Can you work these out from the model? Positions are in its coordinate system, mm. Coordinates: 2 decimals unless noted, no trailing zeros. Order: outer loops, then holes, each group sorted by start corner. A loop starts at its lowest first (then second) coordinate and runs counter-clockwise, first axis right, second up. Notation, with made-up numbers: (13.25, 82) - (70.25, 82) arc R36 cw to (70.25, 118) - close; hole circle Ø7 at (-7, 50). An arc over 180 degrees is marked (long way). Return JSON: item names as keys, results as strings. Group by question number.
1) If I drill on line 1 along Y through (x, z) = (0, -1.15); line 2 along X through (y, z) = (6.5, -1.25); line 3 along Y through (x, z) = (-3.5, -2.6), over which ranges is the centre line in solid material (lowest first)?
2) Imagine slicing it at A-A (y = -20). Write out the boundary of the cut face in (x, z), and give its area (3 significant figures).
3) Imagine slicing it at D-D (y = -10). Write out the boundary of the cut face in (x, z).
4) Imagine slicing it at B-B (z = -0.75). Give the number of separate pieces and of enclosed holes in the cut face, and give its area (3 significant figures).
5) For pin 1 Ø9 at (x, y) = (0, -20) entering from -Z, with a flat end and sliding along its axis, tell me the tip position at first contact or that it passes through.
6) Imagine slicing it at C-C (x = 13). Write out the boundary of the cut face in (y, z), and give its area (3 significant figures).
```python
from build123d import *

# Parameters (mm, degrees)
SM_BASE_FLANGE_1_DEPTH = 3
CUT_EXTRUDE_1_REACH    = 41.166
SKETCH_6_R             = 2.5
CUT_EXTRUDE_2_REACH    = 41.166
SKETCH_7_R             = 5


# Sheet-metal steps are written as plain solids
with BuildPart() as part:
    # Sketch 1 → 基体-法兰1 (new body)
    with BuildSketch(Plane.XY):
        Polygon((20, -30), (14.284239003, -30), (-14.284239003, -30), (-20, -30), (-25, -25), (-25, 21.339745962), (-20, 30), (20, 30), (25, 21.339745962), (25, -25), align=None)
    extrude(amount=-SM_BASE_FLANGE_1_DEPTH)

    # 草图6 → 切除-拉伸1 (cut, up to next)
    with BuildSketch(Plane.XY, mode=Mode.PRIVATE) as cut_extrude_1_sk1:
        with Locations((0, 24)):
            Circle(SKETCH_6_R)
    cut_extrude_1_tool1 = extrude(cut_extrude_1_sk1.sketch, amount=-CUT_EXTRUDE_1_REACH, mode=Mode.PRIVATE) & part.part
    # 草图6 → 切除-拉伸1 (cut, up to next)
    with BuildSketch(Plane.XY, mode=Mode.PRIVATE) as cut_extrude_1_sk2:
        with Locations((-17.8, -10)):
            Circle(SKETCH_6_R)
    cut_extrude_1_tool2 = extrude(cut_extrude_1_sk2.sketch, amount=-CUT_EXTRUDE_1_REACH, mode=Mode.PRIVATE) & part.part
    # 草图6 → 切除-拉伸1 (cut, up to next)
    with BuildSketch(Plane.XY, mode=Mode.PRIVATE) as cut_extrude_1_sk3:
        with Locations((17.8, -10)):
            Circle(SKETCH_6_R)
    cut_extrude_1_tool3 = extrude(cut_extrude_1_sk3.sketch, amount=-CUT_EXTRUDE_1_REACH, mode=Mode.PRIVATE) & part.part
    # 草图6 → 切除-拉伸1 (cut, up to next)
    with BuildSketch(Plane.XY, mode=Mode.PRIVATE) as cut_extrude_1_sk4:
        with Locations((-12.5, 20)):
            Circle(SKETCH_6_R)
    cut_extrude_1_tool4 = extrude(cut_extrude_1_sk4.sketch, amount=-CUT_EXTRUDE_1_REACH, mode=Mode.PRIVATE) & part.part
    # 草图6 → 切除-拉伸1 (cut, up to next)
    with BuildSketch(Plane.XY, mode=Mode.PRIVATE) as cut_extrude_1_sk5:
        with Locations((12.5, 20)):
            Circle(SKETCH_6_R)
    cut_extrude_1_tool5 = extrude(cut_extrude_1_sk5.sketch, amount=-CUT_EXTRUDE_1_REACH, mode=Mode.PRIVATE) & part.part
    add(cut_extrude_1_tool1.solids().sort_by_distance((0, 24, 0))[0], mode=Mode.SUBTRACT)
    add(cut_extrude_1_tool2.solids().sort_by_distance((-17.8, -10, 0))[0], mode=Mode.SUBTRACT)
    add(cut_extrude_1_tool3.solids().sort_by_distance((17.8, -10, 0))[0], mode=Mode.SUBTRACT)
    add(cut_extrude_1_tool4.solids().sort_by_distance((-12.5, 20, 0))[0], mode=Mode.SUBTRACT)
    add(cut_extrude_1_tool5.solids().sort_by_distance((12.5, 20, 0))[0], mode=Mode.SUBTRACT)

    # 草图7 → 切除-拉伸2 (cut, up to next)
    with BuildSketch(Plane.XY, mode=Mode.PRIVATE) as cut_extrude_2_sk1:
        with Locations((-15, 5)):
            Circle(SKETCH_7_R)
    cut_extrude_2_tool1 = extrude(cut_extrude_2_sk1.sketch, amount=-CUT_EXTRUDE_2_REACH, mode=Mode.PRIVATE) & part.part
    # 草图7 → 切除-拉伸2 (cut, up to next)
    with BuildSketch(Plane.XY, mode=Mode.PRIVATE) as cut_extrude_2_sk2:
        with Locations((15, 5)):
            Circle(SKETCH_7_R)
    cut_extrude_2_tool2 = extrude(cut_extrude_2_sk2.sketch, amount=-CUT_EXTRUDE_2_REACH, mode=Mode.PRIVATE) & part.part
    # 草图7 → 切除-拉伸2 (cut, up to next)
    with BuildSketch(Plane.XY, mode=Mode.PRIVATE) as cut_extrude_2_sk3:
        with Locations((0, -20)):
            Circle(SKETCH_7_R)
    cut_extrude_2_tool3 = extrude(cut_extrude_2_sk3.sketch, amount=-CUT_EXTRUDE_2_REACH, mode=Mode.PRIVATE) & part.part
    # 草图7 → 切除-拉伸2 (cut, up to next)
    with BuildSketch(Plane.XY, mode=Mode.PRIVATE) as cut_extrude_2_sk4:
        with Locations((-15, -20)):
            Circle(SKETCH_7_R)
    cut_extrude_2_tool4 = extrude(cut_extrude_2_sk4.sketch, amount=-CUT_EXTRUDE_2_REACH, mode=Mode.PRIVATE) & part.part
    # 草图7 → 切除-拉伸2 (cut, up to next)
    with BuildSketch(Plane.XY, mode=Mode.PRIVATE) as cut_extrude_2_sk5:
        with Locations((15, -20)):
            Circle(SKETCH_7_R)
    cut_extrude_2_tool5 = extrude(cut_extrude_2_sk5.sketch, amount=-CUT_EXTRUDE_2_REACH, mode=Mode.PRIVATE) & part.part
    # 草图7 → 切除-拉伸2 (cut, up to next)
    with BuildSketch(Plane.XY, mode=Mode.PRIVATE) as cut_extrude_2_sk6:
        with Locations((0, 5)):
            Circle(SKETCH_7_R)
    cut_extrude_2_tool6 = extrude(cut_extrude_2_sk6.sketch, amount=-CUT_EXTRUDE_2_REACH, mode=Mode.PRIVATE) & part.part
    add(cut_extrude_2_tool1.solids().sort_by_distance((-15, 5, 0))[0], mode=Mode.SUBTRACT)
    add(cut_extrude_2_tool2.solids().sort_by_distance((15, 5, 0))[0], mode=Mode.SUBTRACT)
    add(cut_extrude_2_tool3.solids().sort_by_distance((0, -20, 0))[0], mode=Mode.SUBTRACT)
    add(cut_extrude_2_tool4.solids().sort_by_distance((-15, -20, 0))[0], mode=Mode.SUBTRACT)
    add(cut_extrude_2_tool5.solids().sort_by_distance((15, -20, 0))[0], mode=Mode.SUBTRACT)
    add(cut_extrude_2_tool6.solids().sort_by_distance((0, 5, 0))[0], mode=Mode.SUBTRACT)


solid = part.part
```
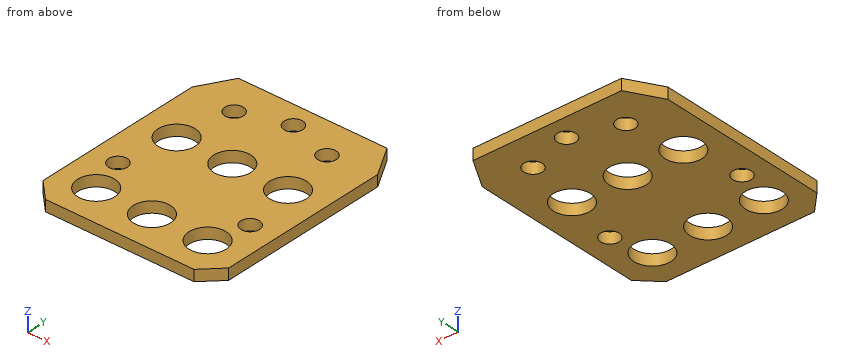
Calculated:
{
 "1": {"line 1": "-30 to -25, -15 to 0, 10 to 21.5, 26.5 to 30", "line 2": "-25 to -19.77, -10.23 to -4.77, 4.77 to 10.23, 19.77 to 25", "line 3": "-30 to -23.57, -16.43 to 1.43, 8.57 to 30"},
 "2": {"outline": "(-25, -3) - (-20, -3) - (-20, 0) - (-25, 0) - close; (-10, -3) - (-5, -3) - (-5, 0) - (-10, 0) - close; (5, -3) - (10, -3) - (10, 0) - (5, 0) - close; (20, -3) - (25, -3) - (25, 0) - (20, 0) - close", "area": "60.0 mm2"},
 "3": {"outline": "(-25, -3) - (-20.3, -3) - (-20.3, 0) - (-25, 0) - close; (-15.3, -3) - (15.3, -3) - (15.3, 0) - (-15.3, 0) - close; (20.3, -3) - (25, -3) - (25, 0) - (20.3, 0) - close"},
 "4": {"separate pieces": "1", "enclosed holes": "11", "area": "2,360 mm2"},
 "5": {"pin 1": "through"},
 "6": {"outline": "(-30, -3) - (-24.58, -3) - (-24.58, 0) - (-30, 0) - close; (-15.42, -3) - (0.42, -3) - (0.42, 0) - (-15.42, 0) - close; (9.58, -3) - (17.55, -3) - (17.55, 0) - (9.58, 0) - close; (22.45, -3) - (30, -3) - (30, 0) - (22.45, 0) - close", "area": "110 mm2"}
}
